Check sheet for the drawn part. Datum: minimum x, y, z corner. Units: mm. Coordinates: 2 decimals unless noted, no trailing zeros. Write each loop counter-clockwise with the first axis right and the second up, starting at its lowest first coordinate (ties: lowest second). Pieces come first, ordered by that corner, then holes. Notation, with made-up numbers: (3, 41.5) -> (24, 41.5) arc R16 ccw to (24, 66.5) -> close; hole circle Ø3 at (67.25, 4.5). An arc over 180 degrees is marked (long way). Answer in a Markdown table with one row per item.
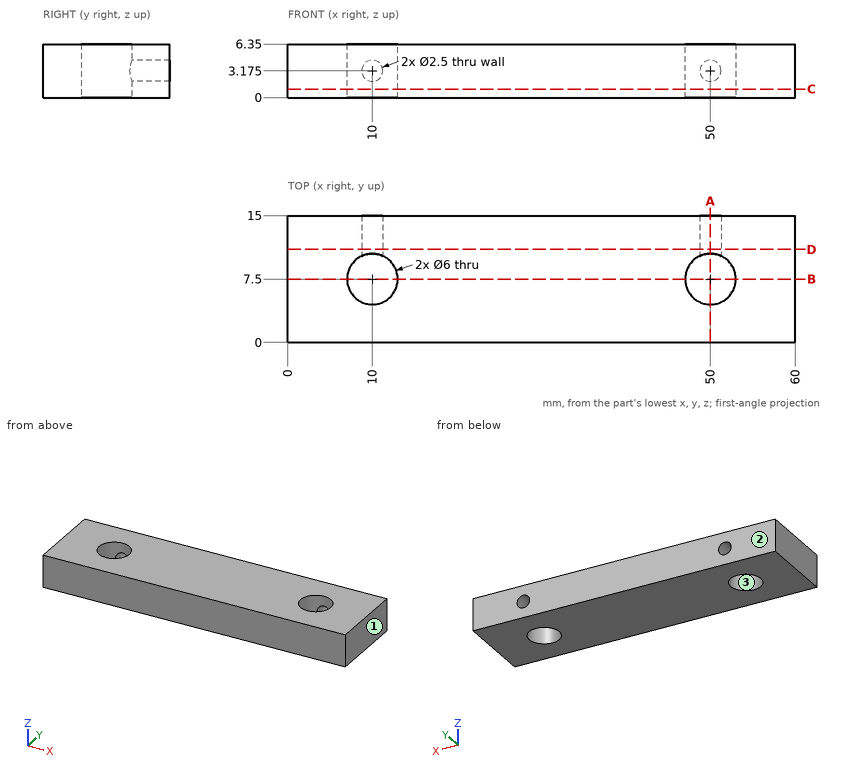
1. Sectioned sample at C-C, the plane z = 1. Record the cut outline in (x, y).
Findings below:
| item | result |
|---|---|
| outline | (0, 0) -> (60, 0) -> (60, 15) -> (0, 15) -> close; hole circle Ø6 at (10, 7.5); hole circle Ø6 at (50, 7.5) |
2. Sectioned sample at A-A, the plane x = 50. Record the cut outline in (y, z) (3 decimals), and give its area (3 significant figures).
Findings below:
| item | result |
|---|---|
| outline | (0, 0) -> (4.5, 0) -> (4.5, 6.35) -> (0, 6.35) -> close; (10.5, 0) -> (15, 0) -> (15, 1.925) -> (10.5, 1.925) -> close; (10.5, 4.425) -> (15, 4.425) -> (15, 6.35) -> (10.5, 6.35) -> close |
| area | 45.9 mm² |
3. Sectioned sample at D-D, the plane y = 11. Record the cut outline in (x, z) (3 decimals).
Findings below:
| item | result |
|---|---|
| outline | (0, 0) -> (60, 0) -> (60, 6.35) -> (0, 6.35) -> close; hole circle Ø2.5 at (10, 3.175); hole circle Ø2.5 at (50, 3.175) |
4. Sectioned sample at B-B, the plane y = 7.5. Record the cut outline in (x, z).
Findings below:
| item | result |
|---|---|
| outline | (0, 0) -> (7, 0) -> (7, 6.35) -> (0, 6.35) -> close; (13, 0) -> (47, 0) -> (47, 6.35) -> (13, 6.35) -> close; (53, 0) -> (60, 0) -> (60, 6.35) -> (53, 6.35) -> close |
5. Go/stop test with a flat-tipped pin: pin 1 (2 mm diameter, centred on x = 50, z = 3.175, fed in from -Y). Record where the tip stops, or that it passes through.
Findings below:
| item | result |
|---|---|
| pin 1 | stops at y = 0 |
6. Material ranges on probe 1 along Z at (x, y) = (50, 11.5) (3 decimals); probe 2 along Y at (x, z) = (10, 4.5); probe 3 along X at (y, z) = (6, 1.5), recorded low to high. Write a range as from..to.
Findings below:
| item | result |
|---|---|
| probe 1 | z = 0..1.925, 4.425..6.35 |
| probe 2 | y = 0..4.5, 10.5..15 |
| probe 3 | x = 0..7.4, 12.6..47.4, 52.6..60 |
7. Release check for a two-part mould opening along X. For the marked faces 1, 2 and 3 record: released by +X, released by -X, zero draft, split by the parting line, or undercut.
Findings below:
| item | result |
|---|---|
| face 1 | released by +X |
| face 2 | zero draft |
| face 3 | undercut |
